from build123d import *
from OCP.BRepFilletAPI import BRepFilletAPI_MakeChamfer

# Parameters (mm, degrees)
EXTRUDE_1_DEPTH     = 1
CHAMFER_1_SIZE      = 10
CHAMFER_1_SIZE2     = 7.071067812
CHAMFER_2_SIZE      = 10
SKETCH_3_R          = 1.6
CUT_EXTRUDE_2_DEPTH = 10
SKETCH_4_W          = 20
SKETCH_4_H          = 100.961940777
EXTRUDE_2_DEPTH     = 1
CHAMFER_3_SIZE      = 10


with BuildPart() as part:
    # 草图1 → 凸台-拉伸1 (new body)
    with BuildSketch(Plane(origin=(0, 0, 0), x_dir=(1, 0, 0), z_dir=(0, 1, 0))):
        Polygon((0, 0), (53.033008589, 0), (53.033008589, 55), (0, 108.033008589), align=None)
    extrude(amount=EXTRUDE_1_DEPTH)

    # 倒角1: one chamfer whose edges measure the first distance from different faces: ONE call of the kernel's chamfer builder (chamfer() names one face for all edges)
    chamfer_1_edges_1 = [part.edges().sort_by_distance(p)[0] for p in [
        (0, 0.5, -108.033008589),
    ]]
    chamfer_1_side_1 = [part.faces().sort_by_distance(p)[0] for p in [
        (26.516504294, 0.5, -81.516504294),
    ]]
    chamfer_1_edges_2 = [part.edges().sort_by_distance(p)[0] for p in [
        (53.033008589, 0.5, 0),
    ]]
    chamfer_1 = BRepFilletAPI_MakeChamfer(part.part.solid().wrapped)
    for e in chamfer_1_edges_1:
        chamfer_1.Add(CHAMFER_1_SIZE, CHAMFER_1_SIZE2, e.wrapped, chamfer_1_side_1[0].wrapped)  # the first distance lies on this face
    for e in chamfer_1_edges_2:
        chamfer_1.Add(CHAMFER_1_SIZE, e.wrapped)
    add(Compound.cast(chamfer_1.Shape()), mode=Mode.REPLACE)

    # 倒角2
    chamfer_2_edges = [part.edges().sort_by_distance(p)[0] for p in [
        (53.033008589, 0.5, -55),
    ]]
    chamfer(chamfer_2_edges, length=CHAMFER_2_SIZE)

    # 草图3 → 切除-拉伸2 (cut)
    with BuildSketch(Plane.XZ):
        with Locations(Location((22.980970389, -77.980970389, 0), (0, 0, 270))):
            Circle(SKETCH_3_R)
        with Locations(Location((48.033008589, -27.5, 0), (0, 0, 270))):
            Circle(SKETCH_3_R)
        with Locations(Location((21.516504294, -5, 0), (0, 0, 270))):
            Circle(SKETCH_3_R)
    extrude(amount=-CUT_EXTRUDE_2_DEPTH, mode=Mode.SUBTRACT)

    # 草图4 → 凸台-拉伸2 (add)
    with BuildSketch(Plane.XZ):
        with Locations((-10, -50.480970389)):
            Rectangle(SKETCH_4_W, SKETCH_4_H)
    extrude(amount=-EXTRUDE_2_DEPTH)

    # 倒角3
    chamfer_3_edges = [part.edges().sort_by_distance(p)[0] for p in [
        (-20, 0.5, 0),
        (-20, 0.5, -100.961940777),
    ]]
    chamfer(chamfer_3_edges, length=CHAMFER_3_SIZE)


solid = part.part
Geometry: final body of the model. Coordinates: model frame, mm. Round coordinates to 2 decimals unless told otherwise and drop trailing zeros. Loops run counter-clockwise (first coordinate to the right, second up) from the corner with the lowest first, then second, coordinate; pieces in that order, holes last. Notation, with made-up numbers: (20.5, -39.75) -> (44.5, -39.75) arc R8 cw to (44.5, -25.75) -> close; hole circle Ø3 at (75.5, 10). An arc over 180 degrees is marked (long way). One line per question, with ' | ' between items. Start each with the question number.
1. Line query: line 1 along Z through (x, y) = (49, 0.2); line 2 along Z through (x, y) = (47, 0.5); line 3 along X through (y, z) = (0.1, -6). Output: solid intervals per line, ascending. Write a range as [from, to].
2. Section A-A on z = -27.5. Output: boundary loops of the cut face in (x, y), and give its area (3 significant figures).
3. Section C-C on z = -5. Output: boundary loops of the cut face in (x, y).
4. Section D-D on x = 9. Output: boundary loops of the cut face in (y, z).
5. Section B-B on y = 0.55. Output: boundary loops of the cut face in (x, z).
6. Contact query for flat-ended pins moving along their axis: pin 1 (3.5 mm diameter, centred on x = 48.03, z = -27.5, fed in from -Y); pin 2 (3 mm diameter, centred on x = 22.98, z = -77.98, fed in from +Y) (3 decimals). Output: stop coordinate, or through.
7. Mould query, pull axis X, two halves, no side actions, for faces 1 (the face through (16, 1, -50)), 2 (the face through (-14.9, 0.5, -4.9)), 3 (the face through (20.1, 0.49, -5.74)), 4 (the face through (23.051, 0.493, -76.383)). Classes: pulls with the +X half, pulls with the -X half, needs draft (parallel to the pull), parting line crosses it, or undercut.
Returned:
1) line 1: z = [-54.74, -28.77], [-26.23, -5.97] | line 2: z = [-59.56, -28.72], [-26.28, -3.97] | line 3: x = [-16, 20.27], [22.77, 49.03]
2) outline: (-20, 0) -> (46.43, 0) -> (46.43, 1) -> (-20, 1) -> close; (49.63, 0) -> (53.03, 0) -> (53.03, 1) -> (49.63, 1) -> close | area: 69.8 mm2
3) outline: (-15, 0) -> (19.92, 0) -> (19.92, 1) -> (-15, 1) -> close; (23.12, 0) -> (48.03, 0) -> (48.03, 1) -> (23.12, 1) -> close
4) outline: (0, -99.03) -> (1, -99.03) -> (1, 0) -> (0, 0) -> close
5) outline: (-20, -90.96) -> (-10, -100.96) -> (7.07, -100.96) -> (45.96, -62.07) -> (53.03, -45) -> (53.03, -10) -> (43.03, 0) -> (-10, 0) -> (-20, -10) -> close; hole circle Ø3.2 at (21.52, -5); hole circle Ø3.2 at (22.98, -77.98); hole circle Ø3.2 at (48.03, -27.5)
6) pin 1: stops at y = 0 | pin 2: passes through
7) face 1: needs draft | face 2: pulls with the -X half | face 3: undercut | face 4: undercut
